```python
from build123d import *

# Parameters (mm, degrees)
ESQUISSE1_W             = 188
ESQUISSE1_H             = 135
BOSS_EXTRU_1_DEPTH      = 10
ESQUISSE2_W             = 12
ESQUISSE2_H             = 71
BOSS_EXTRU_2_DEPTH      = 140
ESQUISSE4_W             = 63
ESQUISSE4_H             = 140
ENL_V_MAT_EXTRU_1_DEPTH = 140
ESQUISSE6_R             = 2
BOSS_EXTRU_3_DEPTH      = 67
ENL_V_MAT_EXTRU_2_DEPTH = 262.635242274
ESQUISSE11_W            = 20
ESQUISSE11_H            = 10
BOSS_EXTRU_4_DEPTH      = 35
ESQUISSE12_R            = 2
BOSS_EXTRU_5_DEPTH      = 20
ESQUISSE13_W            = 20
ESQUISSE13_H            = 10
BOSS_EXTRU_6_DEPTH      = 35
BOSS_EXTRU_7_START      = 20
ESQUISSE14_R            = 2
BOSS_EXTRU_7_DEPTH      = 20
ESQUISSE15_R            = 2
BOSS_EXTRU_8_DEPTH      = 67
ESQUISSE16_R            = 5
BOSS_EXTRU_9_DEPTH      = 13
ESQUISSE17_R            = 5
BOSS_EXTRU_10_DEPTH     = 6


with BuildPart() as part:
    # Esquisse1 → Boss.-Extru.1 (new body)
    with BuildSketch(Plane(origin=(0, 0, 0), x_dir=(1, 0, 0), z_dir=(0, 1, 0))):
        with Locations((94, 67.5)):
            Rectangle(ESQUISSE1_W, ESQUISSE1_H)
    extrude(amount=BOSS_EXTRU_1_DEPTH)

    # Esquisse2 → Boss.-Extru.2 (add)
    with BuildSketch(Plane(origin=(0, 10, 0), x_dir=(1, 0, 0), z_dir=(0, 1, 0))):
        with Locations((56, 67.5)):
            Rectangle(ESQUISSE2_W, ESQUISSE2_H)
    extrude(amount=BOSS_EXTRU_2_DEPTH)

    # Esquisse4 → Enlèv. mat.-Extru.1 (cut)
    with BuildSketch(Plane(origin=(62, 0, 0), x_dir=(0, 0, -1), z_dir=(1, 0, 0))):
        with Locations((67.5, 80)):
            Rectangle(ESQUISSE4_W, ESQUISSE4_H)
    extrude(amount=-ENL_V_MAT_EXTRU_1_DEPTH, mode=Mode.SUBTRACT)

    # Esquisse6 → Boss.-Extru.3 (add)
    with BuildSketch(Plane.XY.offset(-99)):
        with Locations(Location((56, 144, 0), (0, 0, 90))):
            Circle(ESQUISSE6_R)
    extrude(amount=BOSS_EXTRU_3_DEPTH)

    # Esquisse7 → Enlèv. mat.-Extru.2 (cut, through all)
    with BuildSketch(Plane.XY.offset(-32)):
        with BuildLine():
            Line((50, 145.469087673), (50, 152.744377171))
            Line((50, 152.744377171), (62, 152.744377171))
            Line((62, 152.744377171), (62, 145.469087673))
            ThreePointArc((62, 145.469087673), (56, 150.177233895), (50, 145.469087673))
        make_face()
    extrude(amount=-ENL_V_MAT_EXTRU_2_DEPTH, mode=Mode.SUBTRACT)

    # Esquisse11 → Boss.-Extru.4 (add)
    with BuildSketch(Plane.XZ):
        with Locations((94, -5)):
            Rectangle(ESQUISSE11_W, ESQUISSE11_H)
    extrude(amount=BOSS_EXTRU_4_DEPTH)

    # Esquisse12 → Boss.-Extru.5 (add)
    with BuildSketch(Plane.XY):
        with Locations(Location((94, -25, 0), (0, 0, 180))):
            Circle(ESQUISSE12_R)
    extrude(amount=BOSS_EXTRU_5_DEPTH)

    # Esquisse13 → Boss.-Extru.6 (add)
    with BuildSketch(Plane.XZ):
        with Locations((94, -130)):
            Rectangle(ESQUISSE13_W, ESQUISSE13_H)
    extrude(amount=BOSS_EXTRU_6_DEPTH)

    # Esquisse14 → Boss.-Extru.7 (add)
    with BuildSketch(Plane(origin=(0, 0, -135), x_dir=(-1, 0, 0), z_dir=(0, 0, -1)).offset(BOSS_EXTRU_7_START)):
        with Locations((-94, -25)):
            Circle(ESQUISSE14_R)
    extrude(amount=-BOSS_EXTRU_7_DEPTH)

    # Esquisse15 → Boss.-Extru.8 (add)
    with BuildSketch(Plane.XY.offset(-99)):
        with Locations(Location((56, 112, 0), (0, 0, 90))):
            Circle(ESQUISSE15_R)
    extrude(amount=BOSS_EXTRU_8_DEPTH)

    # Esquisse16 → Boss.-Extru.9 (add)
    with BuildSketch(Plane.XY.offset(-99)):
        with Locations(Location((56, 112, 0), (0, 0, 180))):
            Circle(ESQUISSE16_R)
    extrude(amount=BOSS_EXTRU_9_DEPTH)

    # Esquisse17 → Boss.-Extru.10 (add)
    with BuildSketch(Plane(origin=(0, 0, -36), x_dir=(-1, 0, 0), z_dir=(0, 0, -1))):
        with Locations(Location((-56, 144, 0), (0, 0, 270))):
            Circle(ESQUISSE17_R)
    extrude(amount=BOSS_EXTRU_10_DEPTH)


solid = part.part
```
Work out the finished part from the listing and answer in its coordinate system (mm). A direction names the side the tool comes from. Give positions to 0.01 mm unless a question says otherwise; leave off trailing zeros. Write each loop counter-clockwise with the first axis right and the second up, starting at its lowest first coordinate (ties: lowest second). Pieces come first, ordered by that corner, then holes.
(1) The part is cut by section B-B on z = -95. Write down the section's boundary in (x, y).
Final values:
outline: (0, 0) - (188, 0) - (188, 10) - (0, 10) - close; circle Ø10 at (56, 112); circle Ø4 at (56, 144)
(2) The part is cut by section D-D on y = 3. Write down the section's boundary in (x, z).
Final values:
outline: (0, -135) - (188, -135) - (188, 0) - (0, 0) - close
(3) The part is cut by section C-C on x = 125. Write down the section's boundary in (y, z).
Final values:
outline: (0, -135) - (10, -135) - (10, 0) - (0, 0) - close
(4) Flat-ended cylindrical pins translate along their axes: pin 1 Ø8 at (y, z) = (-15.5, -3.5) entering from +X; pin 2 Ø3 at (y, z) = (-19.5, -129.5) entering from -X; pin 3 Ø8 at (x, y) = (57.5, 112.5) entering from +Z; pin 4 Ø3 at (y, z) = (65.5, -105) entering from +X. Find the tip coordinate at first contact, or state that the pin passes through.
Final values:
pin 1: stops at x = 104
pin 2: stops at x = 84
pin 3: stops at z = -32
pin 4: passes through
(5) The part is cut by section A-A on y = 47.5. Write down the section's boundary in (x, z), plus the area to 3 significant figures.
Final values:
outline: (50, -103) - (62, -103) - (62, -99) - (50, -99) - close; (50, -36) - (62, -36) - (62, -32) - (50, -32) - close
area: 96.0 mm2
(6) Straight lines are drawn through the part: line 1 (Y direction, x = 148, z = -25); line 2 (Z direction, x = 140.5, y = 3); line 3 (Z direction, x = 54, y = 68). For each, find the intervals that lie inside material, in ascending order.
Final values:
line 1: y = 0 to 10
line 2: z = -135 to 0
line 3: z = -103 to -99, -36 to -32
(7) Which of the six approach directions +Z, -Z, +X, -X, +Y, -Y give full straight-line access (tool end or side, diameter ignored) to faces 1 (the flat face through (56, 79, -103)), 2 (the flat face through (104, -17, -5)), 3 (the flat face through (58.2, 144.1, -42)), 4 (the flat face through (56, 79, -32))?
Final values:
face 1: -Z, +X, -X, +Y
face 2: +Z, -Z, +X, -Y
face 3: none
face 4: +Z, +X, -X, +Y
